Here's how the part is built. I have some questions about the finished solid (model axes, mm). Face numbers are marked on the shaded views. A direction names the side the tool comes from. Round coordinates to 2 decimals unless told otherwise and drop trailing zeros. Order: outer loops, then holes, each group sorted by start corner. A loop starts at its lowest first (then second) coordinate and runs counter-clockwise, first axis right, second up. Notation, with made-up numbers: (-14.5, 59) - (25.5, 59) arc R15 cw to (25.5, 69) - close; hole circle Ø10 at (-19.5, 73.5). An arc over 180 degrees is marked (long way). Answer as a JSON object with one key per item and string values.
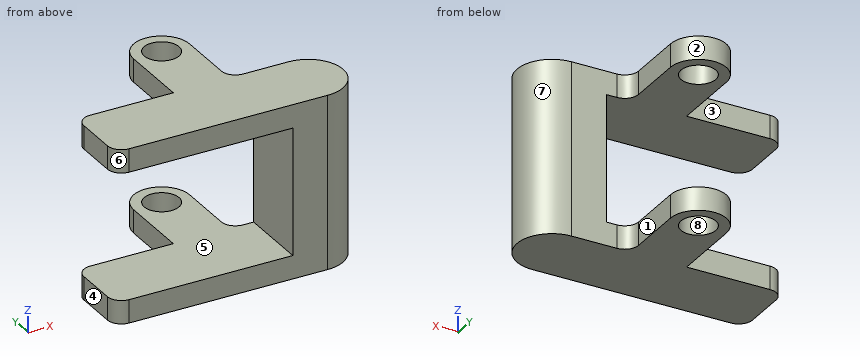
```python
from build123d import *

# Parameters (mm, degrees)
SKETCH1_R           = 18.75
SKETCH1_W           = 104.5375
SKETCH1_H           = 75
BOSS_EXTRUDE1_DEPTH = 25
SKETCH2_R           = 18.75
BOSS_EXTRUDE2_DEPTH = 25
SKETCH3_W           = 75
SKETCH3_H           = 75
BOSS_EXTRUDE3_DEPTH = 136.125
FILLET1_RADIUS      = 37.5
FILLET1_LENGTH      = 186.125
FILLET2_R           = 15


with BuildPart() as part:
    # Sketch1 → Boss-Extrude1 (new body)
    # profile 1 of 3: a face of its own
    with BuildSketch(Plane.XY):
        with BuildLine():
            Line((-986.2125, 179.805377859), (-825, 179.805377859))
            Line((-825, 179.805377859), (-825, 254.805377859))
            Line((-825, 254.805377859), (-926.2125, 254.805377859))
            Line((-926.2125, 254.805377859), (-926.2125, 330.75))
            ThreePointArc((-926.2125, 330.75), (-956.2125, 360.75), (-986.2125, 330.75))
            Line((-986.2125, 330.75), (-986.2125, 254.805377859))
            Line((-986.2125, 254.805377859), (-986.2125, 179.805377859))
        make_face()
        with Locations((-956.2125, 330.75)):
            Circle(SKETCH1_R, mode=Mode.SUBTRACT)
    # profile 2 of 3: a face of its own
    with BuildSketch(Plane.XY):
        with BuildLine():
            Line((-986.2125, 179.805377859), (-825, 179.805377859))
            Line((-825, 179.805377859), (-825, 254.805377859))
            Line((-825, 254.805377859), (-926.2125, 254.805377859))
            Line((-926.2125, 254.805377859), (-926.2125, 330.75))
            ThreePointArc((-926.2125, 330.75), (-956.2125, 360.75), (-986.2125, 330.75))
            Line((-986.2125, 330.75), (-986.2125, 254.805377859))
            Line((-986.2125, 254.805377859), (-986.2125, 179.805377859))
        make_face()
        with Locations((-956.2125, 330.75)):
            Circle(SKETCH1_R, mode=Mode.SUBTRACT)
    # profile 3 of 3: a face of its own
    with BuildSketch(Plane.XY):
        with Locations((-1038.48125, 217.305377859)):
            Rectangle(SKETCH1_W, SKETCH1_H)
    extrude(amount=BOSS_EXTRUDE1_DEPTH)



with BuildPart() as body_2:
    # Sketch2 → Boss-Extrude2 (new body)
    with BuildSketch(Plane(origin=(0, 0, -136.125), x_dir=(-1, 0, 0), z_dir=(0, 0, -1))):
        with BuildLine():
            Line((926.2125, 330.75), (926.2125, 254.805377859))
            Line((926.2125, 254.805377859), (825, 254.805377859))
            Line((825, 254.805377859), (825, 179.805377859))
            Line((825, 179.805377859), (1090.75, 179.805377859))
            Line((1090.75, 179.805377859), (1090.75, 254.805377859))
            Line((1090.75, 254.805377859), (986.2125, 254.805377859))
            Line((986.2125, 254.805377859), (986.2125, 330.75))
            ThreePointArc((986.2125, 330.75), (956.2125, 360.75), (926.2125, 330.75))
        make_face()
        with Locations(Location((956.2125, 330.75, 0), (0, 0, 180))):
            Circle(SKETCH2_R, mode=Mode.SUBTRACT)
    extrude(amount=BOSS_EXTRUDE2_DEPTH)


with BuildPart() as part_1:
    add(part.part)

    add(body_2.part)  # Boss-Extrude3 merges body 2
    # Sketch3 → Boss-Extrude3 (add)
    with BuildSketch(Plane.XY.offset(-136.125)):
        with Locations((-862.5, 217.305377859)):
            Rectangle(SKETCH3_W, SKETCH3_H)
    extrude(amount=BOSS_EXTRUDE3_DEPTH)

    # Fillet1: full round fillet: the end face becomes a half cylinder, R = half its width
    fillet1_face = Plane((-825, 217.305377859, -68.0625), x_dir=(0, 0, 1), z_dir=(1, 0, 0))  # on the end face: x along it, z out of the body
    fillet1_slab = fillet1_face.offset(-FILLET1_RADIUS / 2) * Box(FILLET1_LENGTH, 2 * FILLET1_RADIUS, FILLET1_RADIUS, mode=Mode.PRIVATE)  # the body's end, R deep
    fillet1_round = Plane((-862.5, 217.305377859, -68.0625), x_dir=(1, 0, 0), z_dir=(0, 0, 1)) * Cylinder(FILLET1_RADIUS, FILLET1_LENGTH, mode=Mode.PRIVATE)  # its axis R under the face
    add(fillet1_slab - fillet1_round, mode=Mode.SUBTRACT)

    # Fillet2
    fillet2_edges = [part_1.edges().sort_by_distance(p)[0] for p in [
        (-926.2125, 254.805377859, 12.5),
        (-1090.75, 179.805377859, 12.5),
        (-1090.75, 254.805377859, 12.5),
        (-926.2125, 254.805377859, -148.625),
        (-1090.75, 179.805377859, -148.625),
        (-1090.75, 254.805377859, -148.625),
    ]]
    fillet(fillet2_edges, radius=FILLET2_R)


solid = part_1.part
```
1. Imagine slicing it at A-A (y = 279). List the corners of the cut face in (x, z) for me (1 decimal), plus the area to 3 significant figures.
Responses:
{"outline": "(-986.2, -161.1) - (-926.2, -161.1) - (-926.2, -136.1) - (-986.2, -136.1) - close; (-986.2, 0) - (-926.2, 0) - (-926.2, 25) - (-986.2, 25) - close", "area": "3,000 mm2"}
2. Thinking about a two-plate mould opening in Y: for the marked faces 6, 7 and 8, which applies, pulls with the +Y half, pulls with the -Y half, needs draft (parallel to the pull), parting line crosses it, or undercut?
Responses:
{"face 6": "pulls with the -Y half", "face 7": "parting line crosses it", "face 8": "undercut"}
3. Imagine slicing it at B-B (x = -1038). List the corners of the cut face in (y, z) for me (3 decimals), plus the area to 3 significant figures.
Responses:
{"outline": "(179.805, -161.125) - (254.805, -161.125) - (254.805, -136.125) - (179.805, -136.125) - close; (179.805, 0) - (254.805, 0) - (254.805, 25) - (179.805, 25) - close", "area": "3,750 mm2"}
4. For the marked faces 1, 2, 3, 4 and 5, which set-ups out of +Z, -Z, +X, -X, +Y, -Y let a thin tool reach every point of the face, with its end or its side?
Responses:
{"face 1": "+Z, -Z, +X, +Y", "face 2": "+Z, -Z, +Y", "face 3": "+Z, -Z, -X, +Y", "face 4": "+Z, -Z, -X, +Y, -Y", "face 5": "-X, +Y, -Y"}
5. If I drill on L1, parallel to Z at x = -933.5, y = 280.5 (3 decimals); L2, parallel to X at y = 330.75, z = -154; L3, parallel to X at y = 330, z = -155, over which ranges is the centre line in solid material (lowest first)? Write a range as [from, to].
Responses:
{"L1": "[-161.125, -136.125], [0, 25]", "L2": "[-986.21, -974.96], [-937.46, -926.21]", "L3": "[-986.21, -974.95], [-937.48, -926.21]"}
6. Imagine slicing it at D-D (y = 233.5). List the corners of the cut face in (x, z) for me (3 decimals), plus the area to 3 significant figures.
Responses:
{"outline": "(-1090.75, -161.125) - (-828.677, -161.125) - (-828.677, 25) - (-1090.75, 25) - (-1090.75, 0) - (-900, 0) - (-900, -136.125) - (-1090.75, -136.125) - close", "area": "22,800 mm2"}
7. For P1, Ø24.5, axis at x = -885, z = -105.5, coming from the +Y side; P2, Ø12.5, axis at y = 305.5, z = -151, coming from the -X side; P3, Ø22.5, axis at y = 212.5, z = -92, coming from the -X side, each with a flat end and sliding along its axis, tell me the tip position at first contact or that it passes through.
Responses:
{"P1": "y = 254.81", "P2": "x = -986.21", "P3": "x = -900"}
8. Imagine slicing it at C-C (z = 10). List the corners of the cut face in (x, y) for me, plus the area to 3 significant figures.
Responses:
{"outline": "(-1090.75, 194.81) arc R15 ccw to (-1075.75, 179.81) - (-862.5, 179.81) arc R37.5 ccw to (-862.5, 254.81) - (-911.21, 254.81) arc R15 cw to (-926.21, 269.81) - (-926.21, 330.75) arc R30 ccw to (-986.21, 330.75) - (-986.21, 254.81) - (-1075.75, 254.81) arc R15 ccw to (-1090.75, 239.81) - close; hole circle Ø37.5 at (-956.21, 330.75)", "area": "24,100 mm2"}
